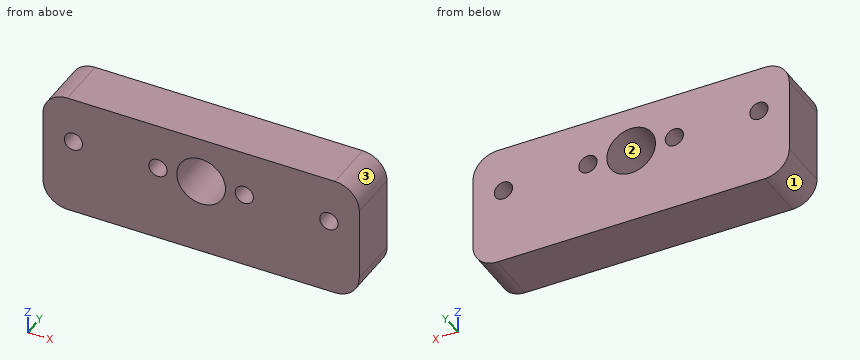
```python
from build123d import *

# Parameters (mm, degrees)
SKETCH1_R           = 4
SKETCH1_R_2         = 1.5
BOSS_EXTRUDE1_DEPTH = 8.6


with BuildPart() as part:
    # Sketch1 → Boss-Extrude1 (new body)
    with BuildSketch(Plane(origin=(0, 0, 0), x_dir=(1, 0, 0), z_dir=(0, 1, 0))):
        with BuildLine():
            Line((-22, 10), (22, 10))
            ThreePointArc((22, 10), (24.828427125, 8.828427125), (26, 6))
            Line((26, 6), (26, -6))
            ThreePointArc((26, -6), (24.828427125, -8.828427125), (22, -10))
            Line((22, -10), (-22, -10))
            ThreePointArc((-22, -10), (-24.828427125, -8.828427125), (-26, -6))
            Line((-26, -6), (-26, 6))
            ThreePointArc((-26, 6), (-24.828427125, 8.828427125), (-22, 10))
        make_face()
        with Locations((0, -2.5)):
            Circle(SKETCH1_R, mode=Mode.SUBTRACT)
        with Locations((7.1, -2.5)):
            Circle(SKETCH1_R_2, mode=Mode.SUBTRACT)
        with Locations((21, -2.5)):
            Circle(SKETCH1_R_2, mode=Mode.SUBTRACT)
        with Locations((-21, -2.5)):
            Circle(SKETCH1_R_2, mode=Mode.SUBTRACT)
        with Locations((-7.1, -2.5)):
            Circle(SKETCH1_R_2, mode=Mode.SUBTRACT)
    extrude(amount=BOSS_EXTRUDE1_DEPTH)


solid = part.part
```
Source: CAD feature listing. Evaluate the final solid. Frame: model axes, mm. Face numbers are marked on the shaded views. Give positions to 0.01 mm unless a question says otherwise; leave off trailing zeros. Order: outer loops, then holes, each group sorted by start corner. A loop starts at its lowest first (then second) coordinate and runs counter-clockwise, first axis right, second up. Notation, with made-up numbers: (-37, -36.75) -> (10, -36.75) arc R19 cw to (10, -11.75) -> close; hole circle Ø7 at (47, 78). An arc over 180 degrees is marked (long way). Use a Markdown table: item, result.
Q1. Material intervals for line 1 (X direction, y = 3.75, z = 2.5); line 2 (Z direction, x = 0, y = 3); line 3 (Z direction, x = -21, y = 5.25), sorted ascending. Write a range as [from, to].
A:
| item | result |
|---|---|
| line 1 | [-26, -22.5], [-19.5, -8.6], [-5.6, -4], [4, 5.6], [8.6, 19.5], [22.5, 26] |
| line 2 | [-10, -1.5], [6.5, 10] |
| line 3 | [-10, 1], [4, 10] |
Q2. Pull-direction query (X, two-part tool) for the marked faces 1, 2 and 3; classes: +X half, -X half, draft (parallel to the pull), parting line (faces both ways), or undercut.
A:
| item | result |
|---|---|
| face 1 | -X half |
| face 2 | undercut |
| face 3 | +X half |
Q3. First-contact query: P1, Ø1, axis at y = 4, z = -7, coming from the -X side; P2, Ø1.8, axis at x = 7.1, z = 2.5, coming from the -Y side. Flat tips, straight axial feed; report the tip coordinate or a pass-through.
A:
| item | result |
|---|---|
| P1 | x = -25.97 |
| P2 | through |
Q4. Section C-C (y = 3). Return the cut outline in (x, z).
A:
| item | result |
|---|---|
| outline | (-26, -6) arc R4 ccw to (-22, -10) -> (22, -10) arc R4 ccw to (26, -6) -> (26, 6) arc R4 ccw to (22, 10) -> (-22, 10) arc R4 ccw to (-26, 6) -> close; hole circle Ø3 at (-21, 2.5); hole circle Ø3 at (-7.1, 2.5); hole circle Ø8 at (0, 2.5); hole circle Ø3 at (7.1, 2.5); hole circle Ø3 at (21, 2.5) |
Q5. Section D-D (x = 0). Return the cut outline in (y, z), and give its area (3 significant figures).
A:
| item | result |
|---|---|
| outline | (0, -10) -> (8.6, -10) -> (8.6, -1.5) -> (0, -1.5) -> close; (0, 6.5) -> (8.6, 6.5) -> (8.6, 10) -> (0, 10) -> close |
| area | 103 mm^2 |
Q6. Section A-A (z = 2.5). Return the cut outline in (x, y), and give its area (3 significant figures).
A:
| item | result |
|---|---|
| outline | (-26, 0) -> (-22.5, 0) -> (-22.5, 8.6) -> (-26, 8.6) -> close; (-19.5, 0) -> (-8.6, 0) -> (-8.6, 8.6) -> (-19.5, 8.6) -> close; (-5.6, 0) -> (-4, 0) -> (-4, 8.6) -> (-5.6, 8.6) -> close; (4, 0) -> (5.6, 0) -> (5.6, 8.6) -> (4, 8.6) -> close; (8.6, 0) -> (19.5, 0) -> (19.5, 8.6) -> (8.6, 8.6) -> close; (22.5, 0) -> (26, 0) -> (26, 8.6) -> (22.5, 8.6) -> close |
| area | 275 mm^2 |
Q7. Section B-B (x = -21). Return the cut outline in (y, z).
A:
| item | result |
|---|---|
| outline | (0, -10) -> (8.6, -10) -> (8.6, 1) -> (0, 1) -> close; (0, 4) -> (8.6, 4) -> (8.6, 10) -> (0, 10) -> close |
